The model under review builds one solid part; all positions refer to its coordinate system, in mm. Give positions to 0.01 mm unless a question says otherwise; leave off trailing zeros. Write each loop counter-clockwise with the first axis right and the second up, starting at its lowest first coordinate (ties: lowest second). Pieces come first, ordered by that corner, then holes. Notation, with made-up numbers: (23.5, 36.25) - (65.5, 36.25) arc R11 ccw to (65.5, 44.25) - close; hole circle Ø4 at (32, 55.25). An arc over 180 degrees is marked (long way). Write item = value, one per line.
```python
from build123d import *

# Parameters (mm, degrees)
SKETCH1_R           = 19.45
SKETCH1_R_2         = 0.75
SKETCH1_R_3         = 3.6
SKETCH1_R_4         = 1.599999975
BOSS_EXTRUDE1_DEPTH = 6


with BuildPart() as part:
    # Sketch1 → Boss-Extrude1 (new body)
    with BuildSketch(Plane.XY):
        with Locations((216.229766611, 107.1388)):
            Circle(SKETCH1_R)
        with Locations((224.322698445, 122.598649751)):
            Circle(SKETCH1_R_2, mode=Mode.SUBTRACT)
        with Locations((222.699474295, 119.497820288)):
            Circle(SKETCH1_R_2, mode=Mode.SUBTRACT)
        with Locations((221.076250145, 116.396990825)):
            Circle(SKETCH1_R_2, mode=Mode.SUBTRACT)
        with Locations((219.453025995, 113.296161362)):
            Circle(SKETCH1_R_2, mode=Mode.SUBTRACT)
        with Locations((231.689616361, 99.045868165)):
            Circle(SKETCH1_R_2, mode=Mode.SUBTRACT)
        with Locations((228.588786898, 100.669092315)):
            Circle(SKETCH1_R_2, mode=Mode.SUBTRACT)
        with Locations((225.487957435, 102.292316466)):
            Circle(SKETCH1_R_2, mode=Mode.SUBTRACT)
        with Locations((222.387127973, 103.915540616)):
            Circle(SKETCH1_R_2, mode=Mode.SUBTRACT)
        with Locations((208.136834776, 91.678950249)):
            Circle(SKETCH1_R_2, mode=Mode.SUBTRACT)
        with Locations((209.760058926, 94.779779712)):
            Circle(SKETCH1_R_2, mode=Mode.SUBTRACT)
        with Locations((211.383283076, 97.880609175)):
            Circle(SKETCH1_R_2, mode=Mode.SUBTRACT)
        with Locations((213.006507226, 100.981438638)):
            Circle(SKETCH1_R_2, mode=Mode.SUBTRACT)
        with Locations((200.76991686, 115.231731835)):
            Circle(SKETCH1_R_2, mode=Mode.SUBTRACT)
        with Locations((203.870746323, 113.608507685)):
            Circle(SKETCH1_R_2, mode=Mode.SUBTRACT)
        with Locations((206.971575786, 111.985283534)):
            Circle(SKETCH1_R_2, mode=Mode.SUBTRACT)
        with Locations((210.072405248, 110.362059384)):
            Circle(SKETCH1_R_2, mode=Mode.SUBTRACT)
        with Locations((216.229766611, 107.1388)):
            Circle(SKETCH1_R_3, mode=Mode.SUBTRACT)
        with Locations((211.717350559, 121.565450451)):
            Circle(SKETCH1_R_4, mode=Mode.SUBTRACT)
    extrude(amount=BOSS_EXTRUDE1_DEPTH)


solid = part.part
```
1. For line 1 (X direction, y = 110, z = 4); line 2 (X direction, y = 104.5, z = 3); line 3 (Y direction, x = 212.5, z = 4.85), list the stretches that pass through material, from the lowest coordinate up. Write a range as from..to.
Findings below:
line_1 = 196.99..209.42, 210.73..214.04, 218.41..235.47
line_2 = 196.96..213.78, 218.68..221.92, 222.86..235.5
line_3 = 88.05..100.43, 101.53..120.17, 122.96..126.23
2. Take a section at B-B on y = 108. Give the boundary of the cut face in (x, z), and give its area (3 significant figures).
Findings below:
outline = (196.8, 0) - (212.73, 0) - (212.73, 6) - (196.8, 6) - close; (219.73, 0) - (235.66, 0) - (235.66, 6) - (219.73, 6) - close
area = 191 mm²
3. Take a section at A-A on x = 217.5. Give the boundary of the cut face in (y, z).
Findings below:
outline = (87.73, 0) - (103.77, 0) - (103.77, 6) - (87.73, 6) - close; (110.51, 0) - (126.55, 0) - (126.55, 6) - (110.51, 6) - close
4. Draft analysis for pull direction X (two halves, no side actions). For faces 1 (the cylindrical face through (211.286, 98.624, 2.958)), 2 (the cylindrical face through (201.89, 120.28, 2.96)), 3 (the flat face through (216, 103, 0)), state which applies: +X half, -X half, draft (parallel to the pull), parting line (faces both ways), or undercut.
Findings below:
face_1 = undercut
face_2 = parting line
face_3 = draft
5. Take a section at D-D on x = 211.5. Give the boundary of the cut face in (y, z), and give its area (3 significant figures).
Findings below:
outline = (88.27, 0) - (97.14, 0) - (97.14, 6) - (88.27, 6) - close; (98.62, 0) - (119.98, 0) - (119.98, 6) - (98.62, 6) - close; (123.15, 0) - (126, 0) - (126, 6) - (123.15, 6) - close
area = 198 mm²
6. Take a section at C-C on z = 1.35. Count the separate pieces of the cut face and the enclosed holes in it, and give its area (3 significant figures).
Findings below:
separate_pieces = 1
enclosed_holes = 18
area = 1,110 mm²
7. Insertion check: P1, Ø3, axis at y = 110.5, z = 2.5, coming from the -X side; P2, Ø1.5, axis at x = 212, z = 2, coming from the -Y side; P3, Ø1, axis at x = 217.5, z = 1, coming from the +Y side. Each pin has a flat end and moves straight along its axis. Give the tip position at first contact, or say it passes through.
Findings below:
P1 = 196.87
P2 = 88
P3 = 126.57
